```python
from build123d import *

# Parameters (mm, degrees)
DODANIE_WYCI_GNI_CIE1_DEPTH = 1
SZKIC2_R                    = 3.15
WYTNIJ_WYCI_GNI_CIE1_DEPTH  = 1


with BuildPart() as part:
    # Szkic1 → Dodanie-wyciągnięcie1 (new body)
    with BuildSketch(Plane.XY):
        with BuildLine():
            Line((-12.5, -6), (-12.5, -16))
            Line((-12.5, -16), (12.5, -16))
            Line((12.5, -16), (12.5, -6))
            Line((12.5, -6), (7.91, -6))
            ThreePointArc((7.91, -6), (6.495786438, -5.414213562), (5.91, -4))
            Line((5.91, -4), (5.91, 5.45))
            Line((5.91, 5.45), (5.91, 39.55))
            Line((5.91, 39.55), (-5.85, 39.55))
            Line((-5.85, 39.55), (-5.85, 5.45))
            Line((-5.85, 5.45), (-5.85, -4))
            ThreePointArc((-5.85, -4), (-6.435786438, -5.414213562), (-7.85, -6))
            Line((-7.85, -6), (-12.5, -6))
        make_face()
    extrude(amount=DODANIE_WYCI_GNI_CIE1_DEPTH)

    # Szkic2 → Wytnij-wyciągnięcie1 (cut)
    with BuildSketch(Plane.XY.offset(1)):
        with Locations((0.03, 31.4)):
            Circle(SZKIC2_R)
    extrude(amount=-WYTNIJ_WYCI_GNI_CIE1_DEPTH, mode=Mode.SUBTRACT)


solid = part.part
```
Can you work these out from the model? Positions are in its coordinate system, mm. A direction names the side the tool comes from. Round coordinates to 2 decimals unless told otherwise and drop trailing zeros. Order: outer loops, then holes, each group sorted by start corner. A loop starts at its lowest first (then second) coordinate and runs counter-clockwise, first axis right, second up.
(1) On a 3-axis mill with a long thin cutter (end or side, diameter ignored), from which of +Z, -Z, +X, -X, +Y, -Y can I reach the whole of each face in a straight line? I mean faces 5 (the face through (5.91, 17.5, 0.5)), 6 (the face through (0, 6, 1)), 7 (the face through (-5.85, 18.1, 0.5)). Say none if no direction works.
Results are:
face 5: +Z, -Z, +X, +Y
face 6: +Z, +X, -X, +Y, -Y
face 7: +Z, -Z, -X, +Y
(2) We'd pull the mould along Y, two halves only. Please class faces 1 (the face through (-0.38, 34.523, 0.507)), 2 (the face through (-10.1, -6, 0.5)), 3 (the face through (-0.2, -16, 0.5)), 4 (the face through (-12.5, -10.9, 0.5)): +Y half, -Y half, draft (parallel to the pull), parting line (faces both ways), or undercut.
Results are:
face 1: undercut
face 2: +Y half
face 3: -Y half
face 4: draft
(3) If we section it at D-D (y = 15): Please give me the cut outline in (x, z), plus the area to 3 significant figures.
Results are:
outline: (-5.85, 0) - (5.91, 0) - (5.91, 1) - (-5.85, 1) - close
area: 11.8 mm2
(4) If I drill on L1, parallel to Y at x = 0.03, z = 0.8; L2, parallel to X at y = 10.5, z = 0.9; L3, parallel to X at y = 31, z = 0.7, over which ranges is the centre line in solid material (lowest first)?
Results are:
L1: y = -16 to 28.25, 34.55 to 39.55
L2: x = -5.85 to 5.91
L3: x = -5.85 to -3.09, 3.15 to 5.91
(5) I'm going to push a flat-ended pin straight in: pin 1 (1 mm diameter, centred on x = -7, y = 2, fed in from -Z). Where does the tip first touch, or does it pass through?
Results are:
pin 1: passes through
(6) If we section it at C-C (x = 0.03): Please give me the cut outline in (y, z).
Results are:
outline: (-16, 0) - (28.25, 0) - (28.25, 1) - (-16, 1) - close; (34.55, 0) - (39.55, 0) - (39.55, 1) - (34.55, 1) - close
(7) If we section it at B-B (z = 0.7): Please give me the cut outline in (x, y), plus the area to 3 significant figures.
Results are:
outline: (-12.5, -16) - (12.5, -16) - (12.5, -6) - (7.91, -6) arc R2 cw to (5.91, -4) - (5.91, 39.55) - (-5.85, 39.55) - (-5.85, -4) arc R2 cw to (-7.85, -6) - (-12.5, -6) - close; hole circle Ø6.3 at (0.03, 31.4)
area: 756 mm2
(8) If we section it at A-A (y = 31.4): Please give me the cut outline in (x, z).
Results are:
outline: (-5.85, 0) - (-3.12, 0) - (-3.12, 1) - (-5.85, 1) - close; (3.18, 0) - (5.91, 0) - (5.91, 1) - (3.18, 1) - close
